Geometry: final body of the model. Coordinates: model frame, mm. Give positions to 0.01 mm unless a question says otherwise; leave off trailing zeros. Write each loop counter-clockwise with the first axis right and the second up, starting at its lowest first coordinate (ties: lowest second). Pieces come first, ordered by that corner, then holes.
from build123d import *

# Parameters (mm, degrees)
SKETCH1_W           = 150
SKETCH1_H           = 65
BOSS_EXTRUDE1_DEPTH = 17.5
CUT_EXTRUDE1_DEPTH  = 66
SKETCH3_W           = 143.142
SKETCH3_H           = 58.142
BOSS_EXTRUDE2_DEPTH = 5
CUT_EXTRUDE2_DEPTH  = 6.5
SKETCH6_W           = 65
SKETCH6_H           = 5.5
CUT_EXTRUDE3_DEPTH  = 10


with BuildPart() as part:
    # Sketch1 → Boss-Extrude1 (new body)
    with BuildSketch(Plane(origin=(0, 0, 0), x_dir=(1, 0, 0), z_dir=(0, 1, 0))):
        Rectangle(SKETCH1_W, SKETCH1_H)
    extrude(amount=BOSS_EXTRUDE1_DEPTH)

    # Sketch2 → Cut-Extrude1 (cut, through all)
    with BuildSketch(Plane.XY.offset(32.5)):
        with BuildLine():
            Line((-4, 8.5), (4, 8.5))
            ThreePointArc((4, 8.5), (5.5, 7), (4, 5.5))
            Line((4, 5.5), (-4, 5.5))
            ThreePointArc((-4, 5.5), (-5.5, 7), (-4, 8.5))
        make_face()
        with BuildLine():
            Line((-41.5, 8.5), (-33.5, 8.5))
            ThreePointArc((-33.5, 8.5), (-32, 7), (-33.5, 5.5))
            Line((-33.5, 5.5), (-41.5, 5.5))
            ThreePointArc((-41.5, 5.5), (-43, 7), (-41.5, 8.5))
        make_face()
        with BuildLine():
            Line((33.5, 8.5), (41.5, 8.5))
            ThreePointArc((41.5, 8.5), (43, 7), (41.5, 5.5))
            Line((41.5, 5.5), (33.5, 5.5))
            ThreePointArc((33.5, 5.5), (32, 7), (33.5, 8.5))
        make_face()
    extrude(amount=-CUT_EXTRUDE1_DEPTH, mode=Mode.SUBTRACT)

    # Sketch3 → Boss-Extrude2 (add)
    with BuildSketch(Plane(origin=(0, 17.5, 0), x_dir=(1, 0, 0), z_dir=(0, 1, 0))):
        Rectangle(SKETCH3_W, SKETCH3_H)
    extrude(amount=BOSS_EXTRUDE2_DEPTH)

    # Sketch4 → Cut-Extrude2 (cut)
    with BuildSketch(Plane(origin=(0, 22.5, 0), x_dir=(1, 0, 0), z_dir=(0, 1, 0))):
        Polygon((-60.950867143, 23.961), (-62.330734287, 21.571), (-60.950867143, 19.181), (-58.191132857, 19.181), (-56.811265713, 21.571), (-58.191132857, 23.961), align=None)
        Polygon((-60.950867143, 8.941), (-62.330734287, 6.551), (-60.950867143, 4.161), (-58.191132857, 4.161), (-56.811265713, 6.551), (-58.191132857, 8.941), align=None)
    extrude(amount=-CUT_EXTRUDE2_DEPTH, mode=Mode.SUBTRACT)

    # Sketch6 → Cut-Extrude3 (cut)
    with BuildSketch(Plane(origin=(0, 22.5, 0), x_dir=(1, 0, 0), z_dir=(0, 1, 0))):
        with Locations((24.071, -21.321)):
            Rectangle(SKETCH6_W, SKETCH6_H)
    extrude(amount=-CUT_EXTRUDE3_DEPTH, mode=Mode.SUBTRACT)


solid = part.part
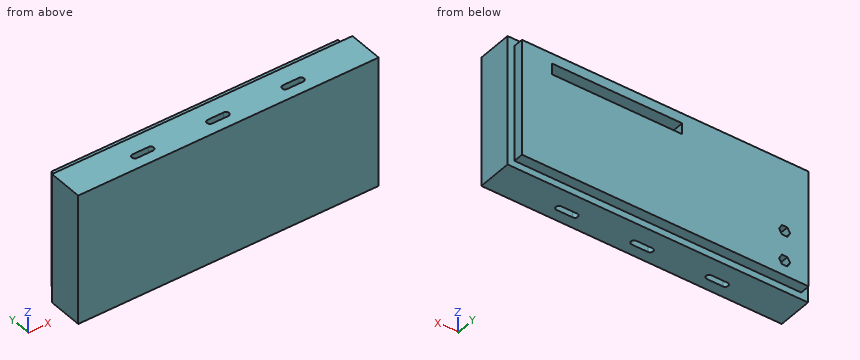
Q1. Section C-C on z = 9.5. Output: boundary loops of the cut face in (x, y).
Filled sheet:
outline: (-75, 0) - (75, 0) - (75, 17.5) - (71.57, 17.5) - (71.57, 22.5) - (-71.57, 22.5) - (-71.57, 17.5) - (-75, 17.5) - close; hole (-41.5, 5.5) - (-33.5, 5.5) arc R1.5 ccw to (-33.5, 8.5) - (-41.5, 8.5) arc R1.5 ccw to start; hole (-4, 5.5) - (4, 5.5) arc R1.5 ccw to (4, 8.5) - (-4, 8.5) arc R1.5 ccw to start; hole (33.5, 5.5) - (41.5, 5.5) arc R1.5 ccw to (41.5, 8.5) - (33.5, 8.5) arc R1.5 ccw to start
Q2. Section D-D on y = 19. Output: boundary loops of the cut face in (x, z).
Filled sheet:
outline: (-71.57, -29.07) - (71.57, -29.07) - (71.57, 29.07) - (-71.57, 29.07) - close; hole (-62.33, -21.57) - (-60.95, -23.96) - (-58.19, -23.96) - (-56.81, -21.57) - (-58.19, -19.18) - (-60.95, -19.18) - close; hole (-62.33, -6.55) - (-60.95, -8.94) - (-58.19, -8.94) - (-56.81, -6.55) - (-58.19, -4.16) - (-60.95, -4.16) - close; hole (-8.43, 18.57) - (56.57, 18.57) - (56.57, 24.07) - (-8.43, 24.07) - close
Q3. Section B-B on x = 0. Output: boundary loops of the cut face in (y, z), plus the area to 3 significant figures.
Filled sheet:
outline: (0, -32.5) - (5.5, -32.5) - (5.5, 32.5) - (0, 32.5) - close; (8.5, -32.5) - (17.5, -32.5) - (17.5, -29.07) - (22.5, -29.07) - (22.5, 18.57) - (12.5, 18.57) - (12.5, 24.07) - (22.5, 24.07) - (22.5, 29.07) - (17.5, 29.07) - (17.5, 32.5) - (8.5, 32.5) - close
area: 1,180 mm2
Q4. Pin query (flat end, axial travel): P1, Ø2, axis at x = -59.5, y = 20, coming from the -Z side; P2, Ø1.5, axis at y = 20.5, z = 4, coming from the -X side; P3, Ø2, axis at x = -60, y = 20, coming from the +Z side. Return the tip coordinate at first contact, or that it passes through.
Filled sheet:
P1: stops at z = -29.07
P2: stops at x = -71.57
P3: stops at z = 29.07
Q5. Section A-A on y = 7. Output: boundary loops of the cut face in (x, z).
Filled sheet:
outline: (-75, -32.5) - (-43, -32.5) - (-43, 32.5) - (-75, 32.5) - close; (-32, -32.5) - (-5.5, -32.5) - (-5.5, 32.5) - (-32, 32.5) - close; (5.5, -32.5) - (32, -32.5) - (32, 32.5) - (5.5, 32.5) - close; (43, -32.5) - (75, -32.5) - (75, 32.5) - (43, 32.5) - close
Q6. Ray query, line 1 along Y through (x, z) = (34, -11.5); line 2 along Z through (x, y) = (11.5, 20.5); line 3 along X through (y, z) = (6.25, 9.5). Return the intervals inside material, ascending.
Filled sheet:
line 1: y = 0 to 5.5, 8.5 to 22.5
line 2: z = -29.07 to 18.57, 24.07 to 29.07
line 3: x = -75 to -42.8, -32.2 to -5.3, 5.3 to 32.2, 42.8 to 75
